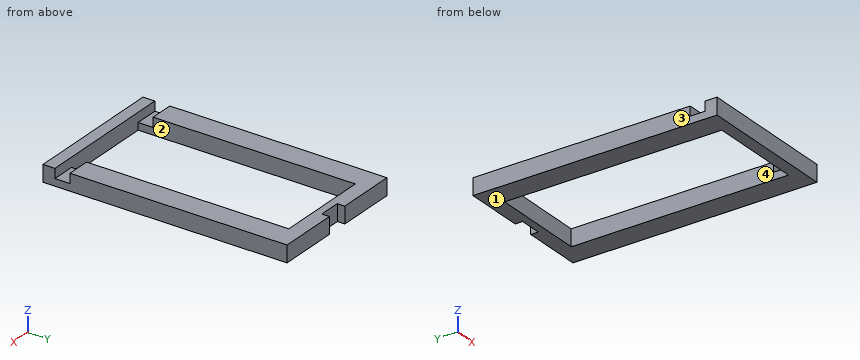
```python
from build123d import *

# Parameters (mm, degrees)
F0_W     = 10
F0_H     = 85
F1_DEPTH = 7
F0_H_2   = 5
F0_H_3   = 6.3
F2_DEPTH = 3


with BuildPart() as f1:
    # F0 (on Top) → F1 (new body)
    with BuildSketch(Plane.XY):
        with Locations((25, 2.5)):
            Rectangle(F0_W, F0_H)
        Polygon((20, 45), (30, 45), (30, 51.3), (4.65, 51.3), (4.65, 48.15), (4.65, 45), align=None)
        Polygon((-30, 45), (-20, 45), (-4.65, 45), (-4.65, 48.15), (-4.65, 51.3), (-30, 51.3), align=None)
        with Locations((-25, 2.5)):
            Rectangle(F0_W, F0_H)
        Polygon((0, 45), (4.65, 45), (4.65, 48.15), (-4.65, 48.15), (-4.65, 45), align=None)
    extrude(amount=F1_DEPTH)



with BuildPart() as f1b:
    # F0 (on Top) → F1, piece 2 (new body)
    with BuildSketch(Plane.XY):
        with Locations((-25, -48.8)):
            Rectangle(F0_W, F0_H_2)
        Polygon((-20, -51.3), (20, -51.3), (20, -46.3), (0, -46.3), (-20, -46.3), align=None)
        with Locations((25, -48.8)):
            Rectangle(F0_W, F0_H_2)
    extrude(amount=F1_DEPTH)


with BuildPart() as f1_1:
    add(f1.part)

    add(f1b.part)  # F2 merges F1b
    # F0 (on Top) → F2 (join)
    with BuildSketch(Plane.XY):
        with Locations((25, -43.15)):
            Rectangle(F0_W, F0_H_3)
        with Locations((-25, -43.15)):
            Rectangle(F0_W, F0_H_3)
    extrude(amount=F2_DEPTH)


solid = f1_1.part
```
Input: part model. Units: mm. Frame: model coordinates. Face numbers are marked on the shaded views. A direction names the side the tool comes from. Coordinates: 2 decimals unless noted, no trailing zeros. Write each loop counter-clockwise with the first axis right and the second up, starting at its lowest first coordinate (ties: lowest second). Pieces come first, ordered by that corner, then holes. Notation, with made-up numbers: M 83.5,51.25 L 104.5,51.25 A14 ccw 104.5,69.25 Z; hole C -5,80.25 d8. An arc over 180 degrees is marked long. Use one line per item in the form item = value.
Q1. Set-up query: the marked faces 3 and 4. Return all of +Z, -Z, +X, -X, +Y, -Y with unobstructed straight access to the full face (end or side cutting, diameter ignored); none if empty.
Answer below:
face_3 = +Z, -Z, -X, +Y, -Y
face_4 = +Z, -Z
Q2. Section B-B (x = -1.5). Return loops of the section in (y, z).
Answer below:
outline = M -51.3,0 L -46.3,0 L -46.3,7 L -51.3,7 Z; M 45,0 L 48.15,0 L 48.15,7 L 45,7 Z
Q3. Section C-C (y = -13.5). Return loops of the section in (x, z), plus the area to 3 significant figures.
Answer below:
outline = M -30,0 L -20,0 L -20,7 L -30,7 Z; M 20,0 L 30,0 L 30,7 L 20,7 Z
area = 140 mm²
Q4. Material intervals for probe 1 along Y at (x, z) = (-6, 5); probe 2 along X at (y, z) = (27, 2.5); probe 3 along Y at (x, z) = (-1.5, 3), sorted ascending. Write a range as from..to.
Answer below:
probe_1 = -51.3..-46.3, 45..51.3
probe_2 = -30..-20, 20..30
probe_3 = -51.3..-46.3, 45..48.15
Q5. Section A-A (z = 4.75). Return loops of the section in (x, y), plus the area to 3 significant figures.
Answer below:
outline = M -30,-51.3 L 30,-51.3 L 30,-46.3 L -30,-46.3 Z; M -30,-40 L -20,-40 L -20,45 L 20,45 L 20,-40 L 30,-40 L 30,51.3 L 4.65,51.3 L 4.65,48.15 L -4.65,48.15 L -4.65,51.3 L -30,51.3 Z
area = 2,350 mm²
Q6. Section D-D (x = 23). Return loops of the section in (y, z), plus the area to 3 significant figures.
Answer below:
outline = M -51.3,0 L 51.3,0 L 51.3,7 L -40,7 L -40,3 L -46.3,3 L -46.3,7 L -51.3,7 Z
area = 693 mm²
Q7. Draft query along Y for the marked faces 1 and 2. Return one class per face: released by +Y, released by -Y, zero draft, split by the parting line, or undercut.
Answer below:
face_1 = zero draft
face_2 = undercut
Q8. First-contact query: pin 1 (1.9 mm diameter, centred on x = -26.5, y = -44.5, fed in from +Z). Flat tip, straight axial feed; report the tip coordinate or a pass-through.
Answer below:
pin_1 = 3
